Could you check a few things on this model? Use its own coordinates, in mm. A direction names the side the tool comes from. Round coordinates to 2 decimals unless told otherwise and drop trailing zeros. Loops run counter-clockwise (first coordinate to the right, second up) from the corner with the lowest first, then second, coordinate; pieces in that order, holes last. Notation, with made-up numbers: (10.25, 87) -> (46.25, 87) arc R25 cw to (46.25, 104) -> close; hole circle Ø4 at (48, 42.5). An arc over 180 degrees is marked (long way). Write each question's results on one line, items separated by ' | '.
from build123d import *

# Parameters (mm, degrees)
SKETCH_1_W              = 22
SKETCH_1_H              = 12
EXTRUDE_1_DEPTH         = 112.2
SKETCH_2_R              = 3
SKETCH_2_W              = 2
SKETCH_2_H              = 6
CUT_EXTRUDE_1_DEPTH     = 116.926010886
SKETCH_3_R              = 1.5
CUT_EXTRUDE_2_DEPTH     = 116.926010886
CUT_EXTRUDE_5_DEPTH     = 116.926010886
HOLE_WIZARD_2_561_D     = 1.778
HOLE_WIZARD_2_561_DEPTH = 1.5
CUT_EXTRUDE_7_DEPTH     = 116.926010886
CUT_EXTRUDE_8_REACH     = 117.926
SKETCH_13_R             = 0.85
CUT_EXTRUDE_START       = 24
CUT_EXTRUDE_9_OUTLINE_R = 0.85
CUT_EXTRUDE_9_DEPTH     = 1
CUT_EXTRUDE_10_DEPTH    = 116.74147918


# Read off the part's stored shape, not the designer's step: Вырез-Вытянуть9
with BuildPart() as part:
    # Эскиз1 → Вытянуть1 (new body)
    with BuildSketch(Plane.XY):
        with BuildLine():
            Line((0.25, 0), (24.75, 0))
            ThreePointArc((24.75, 0), (24.926776695, 0.073223305), (25, 0.25))
            Line((25, 0.25), (25, 14.75))
            ThreePointArc((25, 14.75), (24.926776695, 14.926776695), (24.75, 15))
            Line((24.75, 15), (0.25, 15))
            ThreePointArc((0.25, 15), (0.073223305, 14.926776695), (0, 14.75))
            Line((0, 14.75), (0, 0.25))
            ThreePointArc((0, 0.25), (0.073223305, 0.073223305), (0.25, 0))
        make_face()
        with Locations((12.5, 7.5)):
            Rectangle(SKETCH_1_W, SKETCH_1_H, mode=Mode.SUBTRACT)
    extrude(amount=EXTRUDE_1_DEPTH)

    # Эскиз2 → Вырез-Вытянуть1 (cut, through all)
    with BuildSketch(Plane(origin=(0, 15, 0), x_dir=(1, 0, 0), z_dir=(0, 1, 0))):
        with Locations(Location((12.5, -33.7, 0), (0, 0, 270))):
            Circle(SKETCH_2_R)
        with BuildLine():
            Line((13.560660172, -90.331727984), (4.368272016, -81.139339828))
            ThreePointArc((4.368272016, -81.139339828), (3.636038969, -79.371572875), (4.368272016, -77.603805922))
            Line((4.368272016, -77.603805922), (7.903805922, -74.068272016))
            ThreePointArc((7.903805922, -74.068272016), (9.671572875, -73.336038969), (11.439339828, -74.068272016))
            Line((11.439339828, -74.068272016), (20.631727984, -83.260660172))
            ThreePointArc((20.631727984, -83.260660172), (21.363961031, -85.028427125), (20.631727984, -86.796194078))
            Line((20.631727984, -86.796194078), (17.096194078, -90.331727984))
            ThreePointArc((17.096194078, -90.331727984), (15.328427125, -91.063961031), (13.560660172, -90.331727984))
        make_face()
        with Locations((1, -33.7)):
            Rectangle(SKETCH_2_W, SKETCH_2_H)
        with Locations((24, -33.7)):
            Rectangle(SKETCH_2_W, SKETCH_2_H)
    extrude(amount=-CUT_EXTRUDE_1_DEPTH, mode=Mode.SUBTRACT)

    # Эскиз3 → Вырез-Вытянуть2 (cut, through all)
    with BuildSketch(Plane.ZY):
        with Locations((82.2, 7.5)):
            Circle(SKETCH_3_R)
    extrude(amount=-CUT_EXTRUDE_2_DEPTH, mode=Mode.SUBTRACT)

    # Эскиз6 → Вырез-Вытянуть5 (cut, through all)
    with BuildSketch(Plane(origin=(0, 15, 0), x_dir=(1, 0, 0), z_dir=(0, 1, 0))):
        Polygon((110.629924484, 214.057863156), (10.813103606, 0), (0, -23.188775515), (-99.816820878, -237.246638671), (-527.932547189, -37.612996915), (-317.485801828, 413.691504911), align=None)
    extrude(amount=-CUT_EXTRUDE_5_DEPTH, mode=Mode.SUBTRACT)

    # Эскиз8 → Зенковка для  винта с плоской головкой #2(100)2 (revolve, cut)
    with BuildSketch(Plane(origin=(14.5, 15, 2.5), x_dir=(0, 0, 1), z_dir=(1, 0, 0))):
        Polygon((0, 0), (0, 1.5), (1.35255, 1.5), (1.35255, 0.67945), (2.032, 0), align=None)
    revolve(axis=Axis((14.5, 21.35, 2.5), (0, -1, 0)), mode=Mode.SUBTRACT)

    # Эскиз8 at point 2 (carried to point 2, square into its face) → Зенковка для  винта с плоской головкой #2(100)2 at 2 (revolve, cut)
    with BuildSketch(Plane(origin=(14.5, 0, 2.5), x_dir=(0, 0, 1), z_dir=(-1, 0, 0))):
        Polygon((0, 0), (0, 1.5), (1.35255, 1.5), (1.35255, 0.67945), (2.032, 0), align=None)
    revolve(axis=Axis((14.5, -6.35, 2.5), (0, 1, 0)), mode=Mode.SUBTRACT)

    # Эскиз8 at point 3 (carried to point 3, square into its face) → Зенковка для  винта с плоской головкой #2(100)2 at 3 (revolve, cut)
    with BuildSketch(Plane(origin=(25, 7.5, 2.5), x_dir=(0, 0, 1), z_dir=(0, -1, 0))):
        Polygon((0, 0), (0, 1.5), (1.35255, 1.5), (1.35255, 0.67945), (2.032, 0), align=None)
    revolve(axis=Axis((31.35, 7.5, 2.5), (-1, 0, 0)), mode=Mode.SUBTRACT)

    # Отверстие обработанное метчиком #2-561
    with Locations(Plane.ZY):
        with Locations((27.7, 10.5), (46.2, 2.5)):
            Hole(HOLE_WIZARD_2_561_D / 2, depth=HOLE_WIZARD_2_561_DEPTH)

    # Эскиз12 → Вырез-Вытянуть7 (cut, through all)
    with BuildSketch(Plane.XZ.offset(-15)):
        with BuildLine():
            ThreePointArc((2.791502622, 112.2), (2.947626291, 112.942789468), (3, 113.7))
            ThreePointArc((3, 113.7), (-7.263139721, 116.45), (0.25, 108.936860279))
            Line((0.25, 108.936860279), (0.25, 112.2))
            Line((0.25, 112.2), (2.791502622, 112.2))
        make_face()
        with BuildLine():
            Line((0.25, 112.2), (0.25, 108.936860279))
            ThreePointArc((0.25, 108.936860279), (1.839177493, 110.320423298), (2.791502622, 112.2))
            Line((2.791502622, 112.2), (0.25, 112.2))
        make_face()
    extrude(amount=CUT_EXTRUDE_7_DEPTH, mode=Mode.SUBTRACT)

    # Эскиз13 → Вырез-Вытянуть8 (cut, up to next)
    with BuildSketch(Plane(origin=(25, 0, 0), x_dir=(0, 0, -1), z_dir=(1, 0, 0)), mode=Mode.PRIVATE) as cut_extrude_8_sk1:
        with Locations((-111, 11.5)):
            Circle(SKETCH_13_R)
    cut_extrude_8_tool1 = extrude(cut_extrude_8_sk1.sketch, amount=-CUT_EXTRUDE_8_REACH, mode=Mode.PRIVATE) & part.part
    # Эскиз13 → Вырез-Вытянуть8 (cut, up to next)
    with BuildSketch(Plane(origin=(25, 0, 0), x_dir=(0, 0, -1), z_dir=(1, 0, 0)), mode=Mode.PRIVATE) as cut_extrude_8_sk2:
        with Locations((-111, 3.5)):
            Circle(SKETCH_13_R)
    cut_extrude_8_tool2 = extrude(cut_extrude_8_sk2.sketch, amount=-CUT_EXTRUDE_8_REACH, mode=Mode.PRIVATE) & part.part
    add(cut_extrude_8_tool1.solids().sort_by_distance((25, 11.5, 111))[0], mode=Mode.SUBTRACT)
    add(cut_extrude_8_tool2.solids().sort_by_distance((25, 3.5, 111))[0], mode=Mode.SUBTRACT)

    # Вырез-Вытянуть9 outline → Вырез-Вытянуть9 (cut)
    # profile 1 of 2: a face of its own
    with BuildSketch(Plane.YZ.offset(CUT_EXTRUDE_START)):
        with BuildLine():
            Line((1.8, 112.2), (1.8, 111))
            ThreePointArc((1.8, 111), (3.5, 109.3), (5.2, 111))
            Line((5.2, 111), (5.2, 112.2))
            Line((5.2, 112.2), (1.8, 112.2))
        make_face()
        with Locations((3.5, 111)):
            Circle(CUT_EXTRUDE_9_OUTLINE_R, mode=Mode.SUBTRACT)
    # profile 2 of 2: a face of its own
    with BuildSketch(Plane.YZ.offset(CUT_EXTRUDE_START)):
        with BuildLine():
            Line((13.2, 112.2), (9.8, 112.2))
            Line((9.8, 112.2), (9.8, 111))
            ThreePointArc((9.8, 111), (11.5, 109.3), (13.2, 111))
            Line((13.2, 111), (13.2, 112.2))
        make_face()
        with Locations((11.5, 111)):
            Circle(CUT_EXTRUDE_9_OUTLINE_R, mode=Mode.SUBTRACT)
    extrude(amount=CUT_EXTRUDE_9_DEPTH, mode=Mode.SUBTRACT)

    # Эскиз14 → Вырез-Вытянуть10 (cut, through all)
    with BuildSketch(Plane(origin=(0, 1.5, 0), x_dir=(1, 0, 0), z_dir=(0, 1, 0))):
        with BuildLine():
            Line((-102.051180376, -319.098845535), (17.401923789, -112.2))
            ThreePointArc((17.401923789, -112.2), (20, -110.7), (22.598076211, -112.2))
            Line((22.598076211, -112.2), (142.051180376, -319.098845535))
            Line((142.051180376, -319.098845535), (142.051180376, -796.911262195))
            Line((142.051180376, -796.911262195), (-102.051180376, -796.911262195))
            Line((-102.051180376, -796.911262195), (-102.051180376, -319.098845535))
        make_face()
    extrude(amount=-CUT_EXTRUDE_10_DEPTH, mode=Mode.SUBTRACT)


solid = part.part
1) For faces 1 (the flat face through (12, 1.5, 55)), 2 (the flat face through (1, 8, 30.7)), 3 (the flat face through (24, 3, 110)), 4 (the cylindrical face through (0.76, 2.54, 47.09)), 5 (the flat face through (9.03, 0.76, 85.8)), which set-ups out of +Z, -Z, +X, -X, +Y, -Y let a thin tool reach every point of the face, with its end or its side?
Model answer:
face 1: +Z, -Z | face 2: -X, +Y, -Y | face 3: +Z, +X | face 4: -X | face 5: +Y, -Y
2) If we mould it in two halves opening along Z, with no side actions, what happens to faces 6 (the flat face through (4.23, 13.65, 14.12)), 7 (the flat face through (15.97, 14.26, 78.6)), 8 (the flat face through (25, 7, 74)), 9 (the flat face through (6.11, 0.76, 75.86))? For each: released by +Z, released by -Z, zero draft, split by the parting line, or undercut.
Model answer:
face 6: released by -Z | face 7: undercut | face 8: zero draft | face 9: undercut
3) I want a section at D-D, the plane z = 2.5. Write out the boundary of the cut face in (x, y), plus the area to 3 significant figures.
Model answer:
outline: (9.65, 0) -> (12.47, 0) -> (13.15, 0.68) -> (13.15, 1.5) -> (9.65, 1.5) -> close; (9.65, 13.5) -> (13.15, 13.5) -> (13.15, 14.32) -> (12.47, 15) -> (9.65, 15) -> close; (15.85, 0.68) -> (16.53, 0) -> (24.75, 0) arc R0.25 ccw to (25, 0.25) -> (25, 5.47) -> (24.32, 6.15) -> (23.5, 6.15) -> (23.5, 1.5) -> (15.85, 1.5) -> close; (15.85, 13.5) -> (23.5, 13.5) -> (23.5, 8.85) -> (24.32, 8.85) -> (25, 9.53) -> (25, 14.75) arc R0.25 ccw to (24.75, 15) -> (16.53, 15) -> (15.85, 14.32) -> close | area: 50.5 mm2
4) I need wall thicknesses on line 1 (Y direction, x = 23.95, z = 111); line 2 (X direction, y = 4, z = 50.5); line 3 (Y direction, x = 21.5, z = 63). Which ranges of each line are inside material? Lowest first, please.
Model answer:
line 1: y = 0 to 2.65, 4.35 to 10.65, 12.35 to 15 | line 2: x = 0 to 1.5, 23.5 to 25 | line 3: y = 0 to 1.5, 13.5 to 15
5) I want a section at C-C, the plane x = 5.75. Write out the boundary of the cut face in (y, z).
Model answer:
outline: (0, 10.86) -> (1.5, 10.86) -> (1.5, 76.22) -> (0, 76.22) -> close; (0, 82.52) -> (1.5, 82.52) -> (1.5, 112.2) -> (0, 112.2) -> close; (13.5, 10.86) -> (15, 10.86) -> (15, 76.22) -> (13.5, 76.22) -> close; (13.5, 82.52) -> (15, 82.52) -> (15, 112.2) -> (13.5, 112.2) -> close
6) I want a section at A-A, the plane y = 7.5. Give the number of separate pieces and of enclosed holes in the cut face, plus the area to 3 significant figures.
Model answer:
separate pieces: 7 | enclosed holes: 0 | area: 268 mm2
7) I want a section at B-B, the plane z = 33.7. Write out the boundary of the cut face in (x, y), plus the area to 3 significant figures.
Model answer:
outline: (2, 0) -> (9.5, 0) -> (9.5, 1.5) -> (2, 1.5) -> close; (2, 13.5) -> (9.5, 13.5) -> (9.5, 15) -> (2, 15) -> close; (15.5, 0) -> (23, 0) -> (23, 1.5) -> (15.5, 1.5) -> close; (15.5, 13.5) -> (23, 13.5) -> (23, 15) -> (15.5, 15) -> close | area: 45.0 mm2
8) I'm going to push flat-ended pins straight in: pin 1 (1.6 mm diameter, centred on y = 0.5, z = 32.5, fed in from -X); pin 2 (3 mm diameter, centred on y = 3, z = 111, fed in from +X); pin 3 (1.6 mm diameter, centred on x = 1, y = 7.5, fed in from -Z). Where does each tip first touch, or does it pass through?
Model answer:
pin 1: stops at x = 2 | pin 2: stops at x = 25 | pin 3: stops at z = 19.97
